from build123d import *

# Parameters (mm, degrees)
MODEL_W            = 29
MODEL_H            = 10
MODEL_R            = 0.7
MODEL_W_2          = 2.794
MODEL_H_2          = 1.905
MODEL_W_3          = 1.4
MODEL_H_3          = 1.4
BOSS_EXTRU_1_DEPTH = 1.6


with BuildPart() as part:
    # Model → Boss.-Extru.1 (new body)
    with BuildSketch(Plane.XY):
        with Locations((14.5, 5)):
            Rectangle(MODEL_W, MODEL_H)
        with Locations((26.1, 3.8)):
            Circle(MODEL_R, mode=Mode.SUBTRACT)
        with Locations((26.1, 6.3)):
            Circle(MODEL_R, mode=Mode.SUBTRACT)
        with Locations((26.1, 8.8)):
            Circle(MODEL_R, mode=Mode.SUBTRACT)
        with Locations((2.4, 2.5)):
            Rectangle(MODEL_W_2, MODEL_H_2, mode=Mode.SUBTRACT)
        with BuildLine():
            Line((1.9555, 5.9925), (2.8445, 5.9925))
            ThreePointArc((2.8445, 5.9925), (3.797, 5.04), (2.8445, 4.0875))
            Line((2.8445, 4.0875), (1.9555, 4.0875))
            ThreePointArc((1.9555, 4.0875), (1.003, 5.04), (1.9555, 5.9925))
        make_face(mode=Mode.SUBTRACT)
        with BuildLine():
            Line((1.9555, 8.5325), (2.8445, 8.5325))
            ThreePointArc((2.8445, 8.5325), (3.797, 7.58), (2.8445, 6.6275))
            Line((2.8445, 6.6275), (1.9555, 6.6275))
            ThreePointArc((1.9555, 6.6275), (1.003, 7.58), (1.9555, 8.5325))
        make_face(mode=Mode.SUBTRACT)
        with Locations((26.1, 1.3)):
            Rectangle(MODEL_W_3, MODEL_H_3, mode=Mode.SUBTRACT)
    extrude(amount=BOSS_EXTRU_1_DEPTH)


solid = part.part
CAD build for the part. Positions are in the model's coordinates, mm. A direction names the side the tool comes from. Coordinates: 2 decimals unless noted, no trailing zeros. Write each loop counter-clockwise with the first axis right and the second up, starting at its lowest first coordinate (ties: lowest second). Pieces come first, ordered by that corner, then holes. Notation, with made-up numbers: (59, -16) - (95, -16) arc R9 cw to (95, 0) - close; hole circle Ø11 at (30, 19.25). An arc over 180 degrees is marked (long way). Use a Markdown table: item, result. Add a question column.
Item 1: 3-axis set-ups, long thin cutter, end or side, ignore diameter. For faces 4 (the face through (14, 5, 1.6)), 5 (the face through (2.4, 5.992, 0.8)): which of +Z, -Z, +X, -X, +Y, -Y reach the whole face in a straight line?
Item 2: Band-saw the part on A-A, the plane y = 6.3. Give the cut face in (x, z), and give its area (3 significant figures).
Item 3: Drill centre lines: L1, parallel to Y at x = 26.1, z = 0.95; L2, parallel to X at y = 3, z = 1.05; L3, parallel to X at y = 5.75, z = 1.5. Where is each one in solid material? Low to high. Write a range as from..to.
Item 4: Band-saw the part on C-C, the plane y = 7.5. Give the cut face in (x, z).
Item 5: Band-saw the part on B-B, the plane z = 0.4. Give the cut face in (x, y) (1 decimal).
Item 6: Flat gauge pin, fed straight in: pin 1 (1.1 mm diameter, centred on x = 26.1, y = 6.3, fed in from +Z). Where does the tip first touch, or does it go through?
Item 7: Mould opens along X. For faces 1 (the face through (14, 5, 0)), 2 (the face through (25.4, 3.8, 0.8)), 3 (the face through (29, 5, 1)) say: pulls with the +X half, pulls with the -X half, needs draft (parallel to the pull), parting line crosses it, or undercut.
Numbers:
| question | item | result |
|---|---|---|
| 1 | face 4 | +Z, +X, -X, +Y, -Y |
| 1 | face 5 | +Z, -Z |
| 2 | outline | (0, 0) - (25.4, 0) - (25.4, 1.6) - (0, 1.6) - close; (26.8, 0) - (29, 0) - (29, 1.6) - (26.8, 1.6) - close |
| 2 | area | 44.2 mm2 |
| 3 | L1 | 0..0.6, 2..3.1, 4.5..5.6, 7..8.1, 9.5..10 |
| 3 | L2 | 0..1, 3.8..29 |
| 3 | L3 | 0..1.32, 3.48..25.67, 26.53..29 |
| 4 | outline | (0, 0) - (1.01, 0) - (1.01, 1.6) - (0, 1.6) - close; (3.79, 0) - (29, 0) - (29, 1.6) - (3.79, 1.6) - close |
| 5 | outline | (0, 0) - (29, 0) - (29, 10) - (0, 10) - close; hole (1, 1.5) - (3.8, 1.5) - (3.8, 3.5) - (1, 3.5) - close; hole (2, 4.1) - (2.8, 4.1) arc R1 ccw to (2.8, 6) - (2, 6) arc R1 ccw to start; hole (2, 6.6) - (2.8, 6.6) arc R1 ccw to (2.8, 8.5) - (2, 8.5) arc R1 ccw to start; hole (25.4, 0.6) - (26.8, 0.6) - (26.8, 2) - (25.4, 2) - close; hole circle Ø1.4 at (26.1, 3.8); hole circle Ø1.4 at (26.1, 6.3); hole circle Ø1.4 at (26.1, 8.8) |
| 6 | pin 1 | through |
| 7 | face 1 | needs draft |
| 7 | face 2 | undercut |
| 7 | face 3 | pulls with the +X half |
